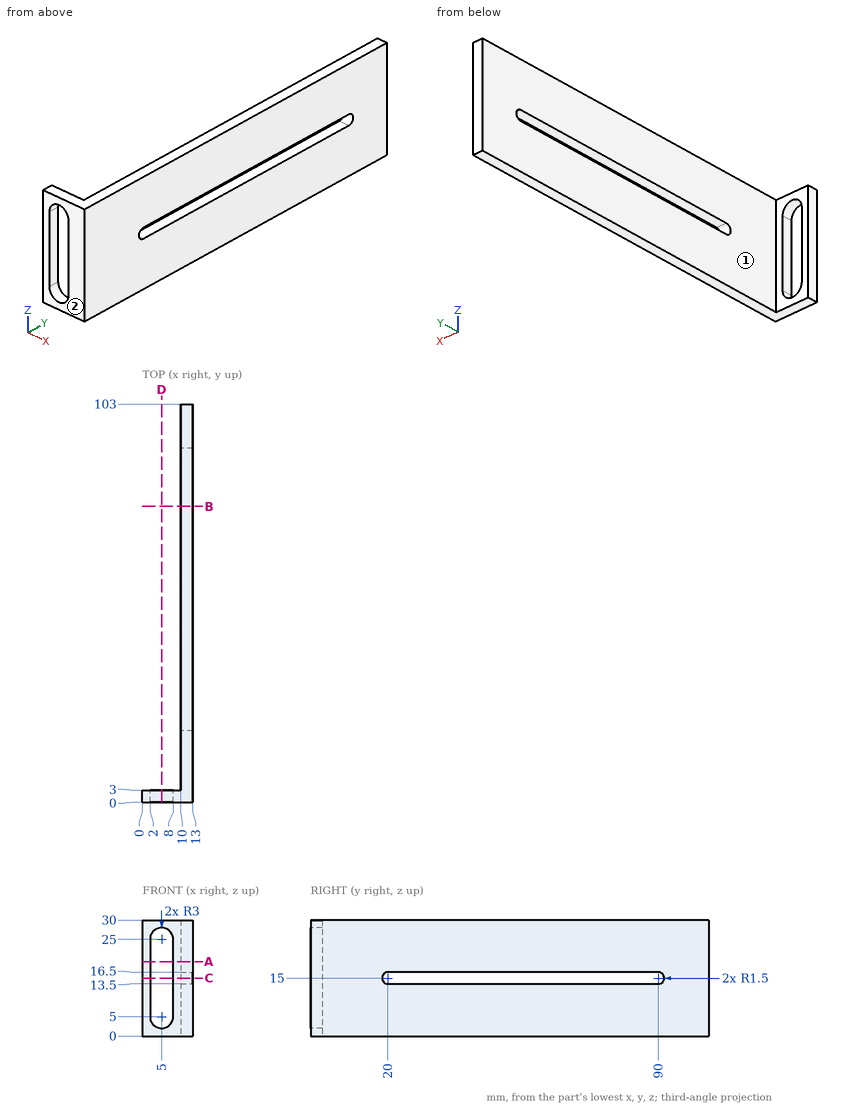
Verification items for this drawing (mm, ordinates from the low corner). A direction names the side the tool comes from. Give positions to 0.01 mm unless a question says otherwise; leave off trailing zeros. Loops run counter-clockwise (first coordinate to the right, second up) from the corner with the lowest first, then second, coordinate; pieces in that order, holes last. Notation, with made-up numbers: M 52.25,52.25 L 57.25,52.25 A20 ccw 57.25,70.25 Z; hole C 11.25,41.25 d2. An arc over 180 degrees is marked long. Answer as a JSON object with one key per item and string values. Group by question number.
Q1. Cross-section at D-D on x = 5. Record the cut outline in (y, z), then the cut area to 3 significant figures.
Q2. Material ranges on line 1 along Z through (x, y) = (12.25, 82.5); line 2 along X through (y, z) = (91.5, 12.25); line 3 along Y through (x, z) = (2.25, 1.5), recorded low to high. Write a range as [from, to].
Q3. Cross-section at B-B on y = 76.5. Record the cut outline in (x, z).
Q4. Cross-section at A-A on z = 19.25. Record the cut outline in (x, y), then the cut area to 3 significant figures.
Q5. Go/stop test with flat-tipped pins: P1, Ø1, axis at y = 84, z = 22, coming from the -X side; P2, Ø6, axis at x = 10, z = 24.5, coming from the -Y side; P3, Ø4, axis at x = 7, z = 5.5, coming from the +Y side. Record where each tip stops, or that it passes through.
Q6. Access from +Z, -Z, +X, -X, +Y, -Y to the whole of each face (thin tool, end or side, straight path). Record for the marked faces 1 and 2.
Q7. Cross-section at C-C on z = 15. Record the cut outline in (x, y), then the cut area to 3 significant figures.
Evaluation:
{
 "1": {"outline": "M 0,0 L 3,0 L 3,2 L 0,2 Z; M 0,28 L 3,28 L 3,30 L 0,30 Z", "area": "12.0 mm2"},
 "2": {"line 1": "z = [0, 13.5], [16.5, 30]", "line 2": "x = [10, 13]", "line 3": "y = [0, 3]"},
 "3": {"outline": "M 10,0 L 13,0 L 13,13.5 L 10,13.5 Z; M 10,16.5 L 13,16.5 L 13,30 L 10,30 Z"},
 "4": {"outline": "M 0,0 L 2,0 L 2,3 L 0,3 Z; M 8,0 L 13,0 L 13,103 L 10,103 L 10,3 L 8,3 Z", "area": "321 mm2"},
 "5": {"P1": "stops at x = 10", "P2": "stops at y = 0", "P3": "stops at y = 3"},
 "6": {"face 1": "+Z, -Z, -X, +Y", "face 2": "+Z, -Z, +X, -X, -Y"},
 "7": {"outline": "M 0,0 L 2,0 L 2,3 L 0,3 Z; M 8,0 L 13,0 L 13,18.5 L 10,18.5 L 10,3 L 8,3 Z; M 10,91.5 L 13,91.5 L 13,103 L 10,103 Z", "area": "102 mm2"}
}
